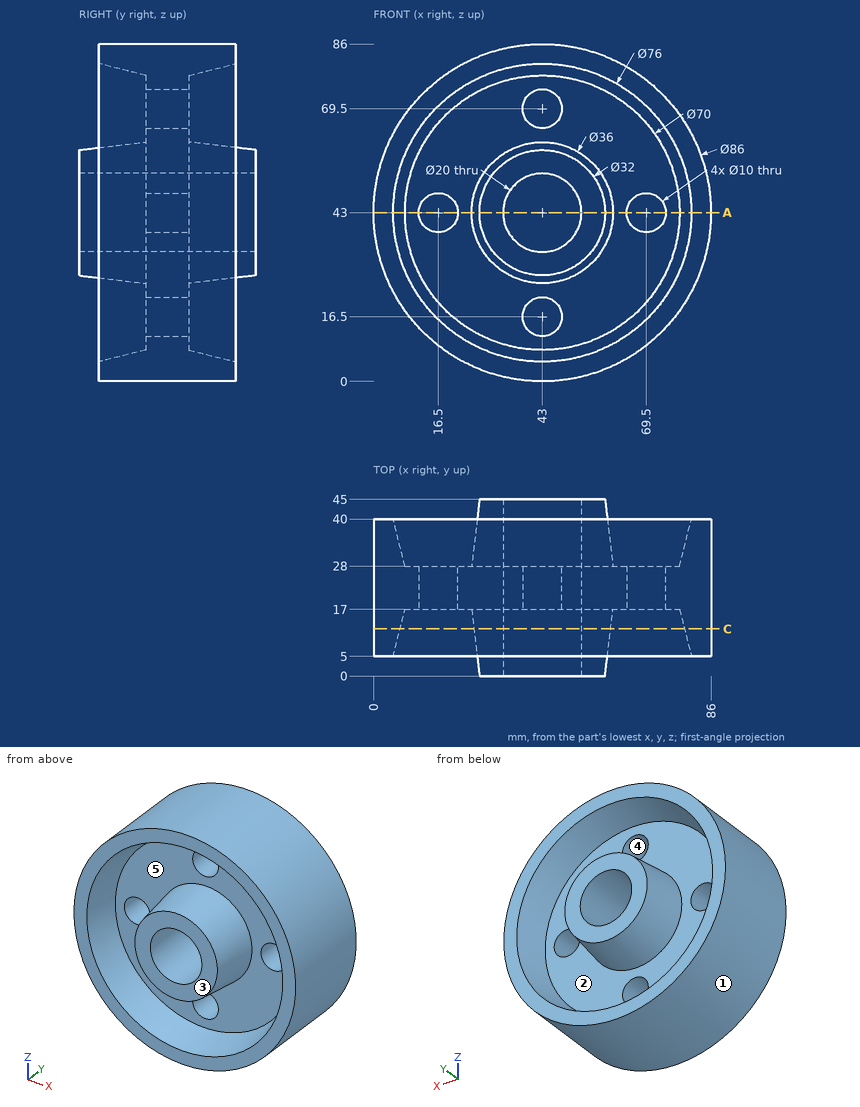
For this review, use the dimensioned drawing (mm, ordinates from the lowest corner) and the shaded views. A direction names the side the tool comes from. Round coordinates to 2 decimals unless told otherwise and drop trailing zeros. Order: outer loops, then holes, each group sorted by start corner. A loop starts at its lowest first (then second) coordinate and runs counter-clockwise, first axis right, second up.
1) Machinability: for the marked faces 4 and 5, which of the approach directions +Z, -Z, +X, -X, +Y, -Y give a long, thin tool a straight path to every point of the face, cutting with its end or side? Answer none if there is none.
The answers:
face 4: +Y, -Y
face 5: -Y
2) Draft analysis for pull direction Z (two halves, no side actions). For the marked faces 1, 2 and 3, state which applies: released by +Z, released by -Z, zero draft, split by the parting line, or undercut.
The answers:
face 1: split by the parting line
face 2: undercut
face 3: zero draft
3) Consider section A-A (z = 43). Count the separate pieces of the cut face and the enclosed holes in it, plus the area to 3 significant figures.
The answers:
separate pieces: 4
enclosed holes: 0
area: 1,290 mm2
4) Consider section C-C (y = 12). State the section outline as (x, z) points.
The answers:
outline: circle Ø86 at (43, 43); circle Ø34.82 at (43, 43); hole circle Ø72.5 at (43, 43); hole circle Ø20 at (43, 43)
5) Clearance check with flat-ended pins moving along their axes: pin 1 Ø13 at (x, z) = (43, 16.5) entering from -Y; pin 2 Ø1 at (x, y) = (13.5, 33.5) entering from +Z; pin 3 Ø10 at (y, z) = (37.5, 70) entering from -X. State where each tip first meets the part, or that it passes through.
The answers:
pin 1: stops at y = 17
pin 2: stops at z = 74.75
pin 3: stops at x = 6.05
6) For L1, parallel to Z at x = 43, y = 22; L2, parallel to Z at x = 42.5, y = 31; L3, parallel to X at y = 12, z = 37.5, list the stretches that pass through material, from the lowest coordinate up.
The answers:
L1: z = 0 to 11.5, 21.5 to 33, 53 to 64.5, 74.5 to 86
L2: z = 0 to 7.25, 25.36 to 33.01, 52.99 to 60.64, 78.75 to 86
L3: x = 0.35 to 7.17, 26.48 to 34.65, 51.35 to 59.52, 78.83 to 85.65
